Verification items for the finished model (mm, model axes). Face numbers are marked on the shaded views. A direction names the side the tool comes from. Round coordinates to 2 decimals unless told otherwise and drop trailing zeros. Loops run counter-clockwise (first coordinate to the right, second up) from the corner with the lowest first, then second, coordinate; pieces in that order, holes last. Notation, with made-up numbers: (20, 68.5) - (68, 68.5) arc R25 cw to (68, 85.5) - close; hole circle Ø10 at (17.5, 51.5). An arc over 180 degrees is marked (long way). Use CSV: the item, a comma, the result in double quotes.
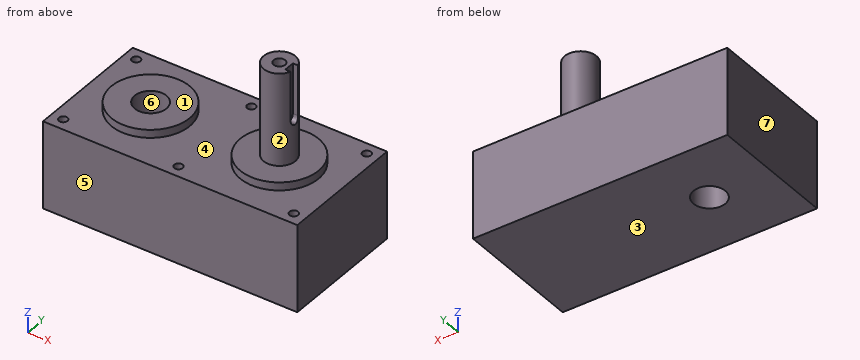
```python
from build123d import *

# Parameters (mm, degrees)
SKETCH1_W                        = 152.4
SKETCH1_H                        = 76.2
BOSS_EXTRUDE1_DEPTH              = 52.324
F_1_4_20_TAPPED_HOLE1_AT_2_COUNT = 2
F_1_4_20_TAPPED_HOLE1_AT_2_PITCH = 69.088
F_1_4_20_TAPPED_HOLE1_AT_3_COUNT = 2
F_1_4_20_TAPPED_HOLE1_AT_3_PITCH = 69.088
SKETCH4_R                        = 23.495
BOSS_EXTRUDE2_DEPTH              = 4.826
SKETCH5_R                        = 9.525
BOSS_EXTRUDE3_DEPTH              = 60.198
CUT_EXTRUDE1_START               = -33.274
CUT_EXTRUDE1_DEPTH               = 33.274
FILLET1_R                        = 3.175
SKETCH7_R                        = 9.525
CUT_EXTRUDE2_DEPTH               = 180.717340566
F_5_16_24_TAPPED_HOLE1_D         = 6.9088
F_5_16_24_TAPPED_HOLE1_DEPTH     = 19.06
F_5_16_24_TAPPED_HOLE1_TIP       = 2.075612922


with BuildPart() as part:
    # Sketch1 → Boss-Extrude1 (new body)
    with BuildSketch(Plane.XY):
        with Locations((76.2, 38.1)):
            Rectangle(SKETCH1_W, SKETCH1_H)
    extrude(amount=BOSS_EXTRUDE1_DEPTH)

    # Sketch2 → 1/4-20 Tapped Hole1 (revolve, cut)
    with BuildSketch(Plane(origin=(76.2, 69.088, 52.324), x_dir=(0, -1, 0), z_dir=(1, 0, 0))):
        Polygon((0, 0), (0, 18.043816902), (2.5527, 16.51), (2.5527, 0), align=None)
    f_1_4_20_tapped_hole1 = revolve(axis=Axis((76.2, 69.088, 58.674), (0, 0, -1)), mode=Mode.SUBTRACT)

    # 1/4-20 Tapped Hole1 at 2: 1/4-20 Tapped Hole1 ×2
    with Locations(*[(-i * F_1_4_20_TAPPED_HOLE1_AT_2_PITCH, 0, 0) for i in range(1, F_1_4_20_TAPPED_HOLE1_AT_2_COUNT)]):
        add(f_1_4_20_tapped_hole1, mode=Mode.SUBTRACT)

    # 1/4-20 Tapped Hole1 at 3: 1/4-20 Tapped Hole1 ×2
    with Locations(*[(i * F_1_4_20_TAPPED_HOLE1_AT_3_PITCH, 0, 0) for i in range(1, F_1_4_20_TAPPED_HOLE1_AT_3_COUNT)]):
        add(f_1_4_20_tapped_hole1, mode=Mode.SUBTRACT)

    # Mirror1: 1/4-20 Tapped Hole1 across plane
    add(f_1_4_20_tapped_hole1.mirror(Plane.ZX.offset(38.1)), mode=Mode.SUBTRACT)

    # Mirror1 copy 1 sketch → Mirror1 copy 1 (revolve, cut)
    with BuildSketch(Plane(origin=(7.112, 7.112, 52.324), x_dir=(0, 1, 0), z_dir=(1, 0, 0))):
        Polygon((0, 0), (0, -18.043816902), (2.5527, -16.51), (2.5527, 0), align=None)
    revolve(axis=Axis((7.112, 7.112, 58.674), (0, 0, 1)), mode=Mode.SUBTRACT)

    # Mirror1 copy 2 sketch → Mirror1 copy 2 (revolve, cut)
    with BuildSketch(Plane(origin=(145.288, 7.112, 52.324), x_dir=(0, 1, 0), z_dir=(1, 0, 0))):
        Polygon((0, 0), (0, -18.043816902), (2.5527, -16.51), (2.5527, 0), align=None)
    revolve(axis=Axis((145.288, 7.112, 58.674), (0, 0, 1)), mode=Mode.SUBTRACT)

    # Sketch4 → Boss-Extrude2 (add)
    with BuildSketch(Plane.XY.offset(52.324)):
        with Locations(Location((37.592, 38.1, 0), (0, 0, 180))):
            Circle(SKETCH4_R)
        with Locations(Location((114.808, 38.1, 0), (0, 0, 180))):
            Circle(SKETCH4_R)
    extrude(amount=BOSS_EXTRUDE2_DEPTH)

    # Sketch5 → Boss-Extrude3 (add)
    with BuildSketch(Plane.XY.offset(52.324)):
        with Locations(Location((114.808, 38.1, 0), (0, 0, 180))):
            Circle(SKETCH5_R)
    extrude(amount=BOSS_EXTRUDE3_DEPTH)

    # Sketch6 → Cut-Extrude1 (cut)
    with BuildSketch(Plane.XY.offset(112.522).offset(CUT_EXTRUDE1_START)):
        with BuildLine():
            Line((120.613256121, 34.925), (120.613256121, 41.275))
            Line((120.613256121, 41.275), (123.788256121, 41.275))
            ThreePointArc((123.788256121, 41.275), (124.333, 38.1), (123.788256121, 34.925))
            Line((123.788256121, 34.925), (120.613256121, 34.925))
        make_face()
    extrude(amount=CUT_EXTRUDE1_DEPTH, mode=Mode.SUBTRACT)

    # Fillet1
    fillet1_edges = [part.edges().sort_by_distance(p)[0] for p in [
        (122.200756121, 41.275, 79.248),
        (122.200756121, 34.925, 79.248),
    ]]
    fillet(fillet1_edges, radius=FILLET1_R - 0.0001)  # a hair under: the kernel refuses the full size

    # Sketch7 → Cut-Extrude2 (cut, through all)
    with BuildSketch(Plane.XY.offset(57.15)):
        with Locations((37.592, 38.1)):
            Circle(SKETCH7_R)
    extrude(amount=-CUT_EXTRUDE2_DEPTH, mode=Mode.SUBTRACT)

    # 5/16-24 Tapped Hole1
    with Locations(Plane.XY.offset(112.522)):
        with Locations((114.808, 38.1)):
            Hole(F_5_16_24_TAPPED_HOLE1_D / 2, depth=F_5_16_24_TAPPED_HOLE1_DEPTH)
            with Locations((0, 0, -(F_5_16_24_TAPPED_HOLE1_DEPTH + F_5_16_24_TAPPED_HOLE1_TIP / 2))):  # 118° drill point
                Cone(0, F_5_16_24_TAPPED_HOLE1_D / 2, F_5_16_24_TAPPED_HOLE1_TIP, mode=Mode.SUBTRACT)


solid = part.part
```
1) Cross-section at A-A, the plane z = 13. Record the cut outline in (x, y) (3 decimals), then the cut area to 3 significant figures.
Returned:
outline,"(0, 0) - (152.4, 0) - (152.4, 76.2) - (0, 76.2) - close; hole circle Ø19.05 at (37.592, 38.1)"
area,"11,300 mm²"
2) Cross-section at D-D, the plane z = 69.5. Record the cut outline in (x, y) (3 decimals), then the cut area to 3 significant figures.
Returned:
outline,"circle Ø19.05 at (114.808, 38.1)"
area,"285 mm²"
3) Mould release check, pull along X, two halves, no side actions. Record for the marked faces 4, 5, 6 and 7: +X half, -X half, draft (parallel to the pull), parting line (faces both ways), or undercut.
Returned:
face 4,"undercut"
face 5,"draft"
face 6,"undercut"
face 7,"-X half"
4) Gauge pin test, flat ends, axial feed: pin 1 Ø11.5 at (x, y) = (37.592, 38.1) entering from -Z; pin 2 Ø23 at (x, y) = (75.5, 47) entering from +Z; pin 3 Ø3 at (x, y) = (7.112, 7.112) entering from +Z; pin 4 Ø3.5 at (x, z) = (122.5, 102.5) entering from -Y. Record the tip position at first contact, or that the pin passes through.
Returned:
pin 1,"passes through"
pin 2,"stops at z = 52.32"
pin 3,"stops at z = 35.18"
pin 4,"stops at y = 30.66"
5) Cross-section at B-B, the plane x = 108.5. Record the cut outline in (y, z), then the cut area to 3 significant figures.
Returned:
outline,"(0, 0) - (76.2, 0) - (76.2, 52.32) - (60.73, 52.32) - (60.73, 57.15) - (45.24, 57.15) - (45.24, 112.52) - (30.96, 112.52) - (30.96, 57.15) - (15.47, 57.15) - (15.47, 52.32) - (0, 52.32) - close"
area,"5,000 mm²"
6) Access from +Z, -Z, +X, -X, +Y, -Y to the whole of each face (thin tool, end or side, straight path). Record for the marked faces 1, 2 and 3.
Returned:
face 1,"+Z, -X, +Y, -Y"
face 2,"+Z"
face 3,"-Z, +X, -X, +Y, -Y"
7) Cross-section at C-C, the plane y = 26. Record the cut outline in (x, z), then the cut area to 3 significant figures.
Returned:
outline,"(0, 0) - (152.4, 0) - (152.4, 52.32) - (134.95, 52.32) - (134.95, 57.15) - (94.67, 57.15) - (94.67, 52.32) - (57.73, 52.32) - (57.73, 57.15) - (17.45, 57.15) - (17.45, 52.32) - (0, 52.32) - close"
area,"8,360 mm²"
8) Thickness scan on probe 1 along X at (y, z) = (67.5, 41); probe 2 along Z at (x, y) = (93, 8.5); probe 3 along X at (y, z) = (56.5, 55). Record the ranges inside material, lowest first. Write a range as [from, to].
Returned:
probe 1,"x = [0, 5.11], [9.11, 74.2], [78.2, 143.29], [147.29, 152.4]"
probe 2,"z = [0, 52.32]"
probe 3,"x = [22.98, 52.2], [100.2, 129.42]"
